from build123d import *

# Parameters (mm, degrees)
SKETCH1_R           = 5.00368331
BOSS_EXTRUDE1_DEPTH = 5


with BuildPart() as part:
    # Sketch1 → Boss-Extrude1 (new, symmetric)
    with BuildSketch(Plane.XY):
        with BuildLine():
            Line((-52.418935372, 39.017679889), (-22.418935372, 39.017679889))
            Line((-22.418935372, 39.017679889), (-22.418935372, 9.017679889))
            Line((-22.418935372, 9.017679889), (-52.418935372, 9.017679889))
            ThreePointArc((-52.418935372, 9.017679889), (-67.418935372, 24.017679889), (-52.418935372, 39.017679889))
        make_face()
        with Locations((-52.418935372, 24.017679889)):
            Circle(SKETCH1_R, mode=Mode.SUBTRACT)
    extrude(amount=BOSS_EXTRUDE1_DEPTH, both=True)

    # Sketch2 → Revolve4 (revolve)
    with BuildSketch(Plane.XY, mode=Mode.PRIVATE) as revolve4_sk:
        Polygon((-22.418935372, 24.017679889), (-22.418935372, 45.324269268), (-15.62342474, 45.324269268), (-15.62342474, 39.194903503), (228.633930204, 39.194903503), (228.633930204, 24.017679889), align=None)
    revolve(revolve4_sk.sketch.rotate(Axis((228.633930204, 24.017679889, 0), (-1, 0, 0)), 90), axis=Axis((228.633930204, 24.017679889, 0), (-1, 0, 0)))


solid = part.part
Work out the finished part from the listing and answer in its coordinate system (mm). A direction names the side the tool comes from. Give positions to 0.01 mm unless a question says otherwise; leave off trailing zeros. Loops run counter-clockwise (first coordinate to the right, second up) from the corner with the lowest first, then second, coordinate; pieces in that order, holes last. Notation, with made-up numbers: (15.25, 41) -> (69.25, 41) arc R15 cw to (69.25, 52) -> close; hole circle Ø6 at (-16, -25.5). An arc over 180 degrees is marked (long way). Use a Markdown table: item, result. Add a question column.
1. For faces 5 (the flat face through (-38, 39.018, 0)), 6 (the flat face through (-45, 24, 5)), 7 (the flat face through (-15.623, 19, 15)), 8 (the flat face through (-45, 24, -5)), 9 (the flat face through (-37, 9.018, 0)), determine the directions among +Z, -Z, +X, -X, +Y, -Y from which every point of the face is accessible in a straight line to the end or side of a thin tool.
2. Section A-A on y = 33 is taken. Determine the outline of the cut face in (x, z).
3. Find the intervals of material crossed by probe 1 along X at (y, z) = (39.5, -10.5); probe 2 along X at (y, z) = (21, 2); probe 3 along X at (y, z) = (15, 8), in increasing order.
4. Section D-D on y = 11.5 is taken. Determine the outline of the cut face in (x, z).
5. Determine the mould class of faces 1 (the cylindrical face through (108.22, 8.97, 1.98)), 2 (the cylindrical face through (-56.107, 27.399, -0.07)), 3 (the cylindrical face through (-67.415, 23.688, 0.07)), 4 (the flat face through (228.634, 24, 0)) for opening direction X: released by +X, released by -X, zero draft, split by the parting line, or undercut.
6. Section B-B on z = 11 is taken. Determine the outline of the cut face in (x, y).
7. Flat-ended cylindrical pins translate along their axes: pin 1 Ø3 at (x, z) = (-38.5, 0) entering from +Y; pin 2 Ø8 at (x, z) = (-25, -15.5) entering from +Y; pin 3 Ø13 at (x, y) = (-52.42, 24.02) entering from -Z. Find the tip coordinate at first contact, or state that the pin passes through.
8. Section C-C on z = 0 is taken. Determine the outline of the cut face in (x, y).
Results below:
| question | item | result |
|---|---|---|
| 1 | face 5 | +Z, -Z, -X, +Y |
| 1 | face 6 | +Z, -X, +Y, -Y |
| 1 | face 7 | +X |
| 1 | face 8 | -Z, -X, +Y, -Y |
| 1 | face 9 | +Z, -Z, -X, -Y |
| 2 | outline | (-64.43, -5) -> (-22.42, -5) -> (-22.42, -19.32) -> (-15.62, -19.32) -> (-15.62, -12.23) -> (228.63, -12.23) -> (228.63, 12.23) -> (-15.62, 12.23) -> (-15.62, 19.32) -> (-22.42, 19.32) -> (-22.42, 5) -> (-64.43, 5) -> close |
| 3 | probe 1 | x = -22.42 to -15.62 |
| 3 | probe 2 | x = -67.11 to -56.41, -48.43 to 228.63 |
| 3 | probe 3 | x = -22.42 to 228.63 |
| 4 | outline | (-60.68, -5) -> (-22.42, -5) -> (-22.42, -17.24) -> (-15.62, -17.24) -> (-15.62, -8.58) -> (228.63, -8.58) -> (228.63, 8.58) -> (-15.62, 8.58) -> (-15.62, 17.24) -> (-22.42, 17.24) -> (-22.42, 5) -> (-60.68, 5) -> close |
| 5 | face 1 | zero draft |
| 5 | face 2 | undercut |
| 5 | face 3 | released by -X |
| 5 | face 4 | released by +X |
| 6 | outline | (-22.42, 5.77) -> (-15.62, 5.77) -> (-15.62, 13.56) -> (228.63, 13.56) -> (228.63, 34.47) -> (-15.62, 34.47) -> (-15.62, 42.27) -> (-22.42, 42.27) -> close |
| 7 | pin 1 | stops at y = 39.02 |
| 7 | pin 2 | stops at y = 41.31 |
| 7 | pin 3 | stops at z = -5 |
| 8 | outline | (-52.42, 9.02) -> (-22.42, 9.02) -> (-22.42, 2.71) -> (-15.62, 2.71) -> (-15.62, 8.84) -> (228.63, 8.84) -> (228.63, 39.19) -> (-15.62, 39.19) -> (-15.62, 45.32) -> (-22.42, 45.32) -> (-22.42, 39.02) -> (-52.42, 39.02) arc R15 ccw to start; hole circle Ø10.01 at (-52.42, 24.02) |
